Check sheet for the modelled part. Datum: model origin and axes. Units: mm. Face numbers are marked on the shaded views. Give positions to 0.01 mm unless a question says otherwise; leave off trailing zeros. Loops run counter-clockwise (first coordinate to the right, second up) from the corner with the lowest first, then second, coordinate; pieces in that order, holes last. Notation, with made-up numbers: (-15, 25.25) -> (34, 25.25) arc R23 cw to (34, 64.25) -> close; hole circle Ø6 at (87.5, 10.25). An arc over 180 degrees is marked (long way). Answer as CSV lines item,"result". Start each with the question number.
(1) Release check for a two-part mould opening along Z. For the marked faces 1, 2 and 3 record: pulls with the +Z half, pulls with the -Z half, needs draft (parallel to the pull), parting line crosses it, or undercut.
(2) Section check A-A on x = 16.5. Enter the section's corners in (y, z).
(3) Section check B-B on z = 7.25. Enter the section's corners in (x, y).
(4) Material ranges on line 1 (Z direction, x = 18.5, y = 1.75); line 2 (X direction, y = 4, z = 4.5); line 3 (Z direction, x = 2.25, y = 0.25), recorded low to high. Write a range as from..to.
from build123d import *

# Parameters (mm, degrees)
BOSS_EXTRUDE1_DEPTH = 7
SKETCH2_W           = 25.128147065
SKETCH2_H           = 19.783027292
BOSS_EXTRUDE2_DEPTH = 2


with BuildPart() as part:
    # Sketch1 → Boss-Extrude1 (new body)
    with BuildSketch(Plane(origin=(0, 0, 0), x_dir=(1, 0, 0), z_dir=(0, 1, 0))):
        Polygon((19.500000402, -8.500000462), (21.50000073, -8.500000462), (21.50000073, 1.499999315), (21.50000073, 1.699998975), (21.467199549, 2.011898905), (21.370301023, 2.31009908), (21.213499829, 2.58169882), (21.003700793, 2.814698964), (20.750001073, 2.998998389), (20.463500172, 3.126598895), (20.156800747, 3.191798925), (19.843200222, 3.191798925), (19.536500797, 3.126598895), (19.249999896, 2.998998389), (18.996300176, 2.814698964), (18.786501139, 2.58169882), (18.670000136, 2.379998565), (11.050600559, 2.379998565), (11.033799499, 2.398598939), (10.99999994, 2.423198894), (10.961800814, 2.440199256), (10.920900851, 2.448899671), (10.879099369, 2.448899671), (10.838199407, 2.440199256), (10.80000028, 2.423198894), (10.766200721, 2.398598939), (10.738201439, 2.367598936), (10.717000812, 2.33049877), (5.719300359, 0), (0, 0), (0, 8.374300694), (25.128147065, 8.374300694), (25.128147065, -11.408726598), (0, -11.408726598), (0, -0.75000152), (1.000002027, -0.75000152), (1.000002027, -1.500001177), (2.000000328, -1.500001177), (2.000000328, -0.75000152), (2.999998629, -0.75000152), (2.999998629, -1.500001177), (4.000000656, -1.500001177), (4.000000656, -0.75000152), (4.999998957, -0.75000152), (4.999998957, -1.500001177), (6.000000983, -1.500001177), (6.000000983, -0.696601346), (6.660599262, -0.388601795), (6.977502257, -1.068301499), (7.883802056, -0.645700842), (7.566899061, 0.033998862), (8.473198861, 0.456599519), (8.790101856, -0.223100185), (9.696502239, 0.199498609), (9.379498661, 0.879198313), (10.285802186, 1.301899552), (10.602802038, 0.622099265), (11.155799031, 0.87999925), (11.199999601, 0.900598243), (11.509099975, 1.044699922), (11.236201972, 1.629998907), (12.199999765, 1.629998907), (12.199999765, 0.87999925), (13.199999928, 0.87999925), (13.199999928, 1.629998907), (14.200000092, 1.629998907), (14.200000092, 0.87999925), (15.200000256, 0.87999925), (15.200000256, 1.629998907), (16.20000042, 1.629998907), (16.20000042, 0.87999925), (17.200000584, 0.87999925), (17.200000584, 1.629998907), (18.200000748, 1.629998907), (18.200000748, 0.87999925), (18.750900403, 0.87999925), (18.786501139, 0.81829913), (18.996300176, 0.585298985), (19.249999896, 0.400999561), (19.500000402, 0.289699063), align=None)
    extrude(amount=BOSS_EXTRUDE1_DEPTH)

    # Sketch2 → Boss-Extrude2 (add)
    with BuildSketch(Plane.XZ):
        with Locations((12.564073533, 1.517212952)):
            Rectangle(SKETCH2_W, SKETCH2_H)
    extrude(amount=BOSS_EXTRUDE2_DEPTH)


solid = part.part
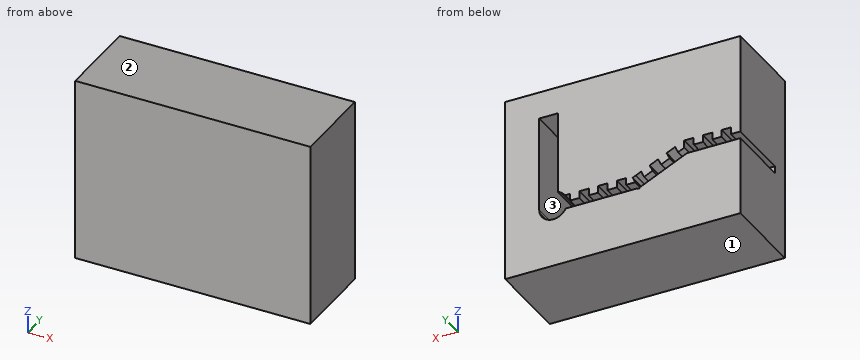
Working result:
1,face 1,"pulls with the -Z half"
1,face 2,"pulls with the +Z half"
1,face 3,"undercut"
2,outline,"(-2, -8.37) -> (7, -8.37) -> (7, -2.38) -> (0, -2.38) -> (0, -0.88) -> (7, -0.88) -> (7, 11.41) -> (-2, 11.41) -> close"
3,outline,"(0, -2) -> (25.13, -2) -> (25.13, 7) -> (21.5, 7) -> (21.5, 0) -> (19.5, 0) -> (19.5, 7) -> (0, 7) -> close"
4,line 1,"z = -8.37..-2.38, -0.88..11.41"
4,line 2,"x = 0..19.5, 21.5..25.13"
4,line 3,"z = -8.37..0, 0.75..11.41"
